```python
from build123d import *

# Parameters (mm, degrees)
BOSS_EXTRUDE1_DEPTH     = 10
CUT_EXTRUDE2_DEPTH      = 50.456381745
CUT_EXTRUDE2_DEPTH_BACK = 50.456381745
SKETCH3_R               = 2.5
CUT_EXTRUDE3_DEPTH      = 6
SKETCH4_R               = 2
CUT_REVOLVE1_ANGLE      = 90
SKETCH5_R               = 2
CUT_EXTRUDE4_DEPTH      = 2.805452299
FILLET1_R               = 5
SKETCH6_W               = 10
SKETCH6_H               = 29.685485307
CUT_EXTRUDE5_DEPTH      = 33
SKETCH7_W               = 19.76767366
SKETCH7_H               = 10
CUT_EXTRUDE6_DEPTH      = 48.418220859
SKETCH8_W               = 3.5
SKETCH8_H               = 11.210857043
CUT_EXTRUDE7_DEPTH      = 48.41822072
FILLET2_R               = 3


with BuildPart() as part:
    # Sketch1 → Boss-Extrude1 (new body)
    with BuildSketch(Plane.XY):
        with BuildLine():
            Line((0, 0), (45, 0))
            Line((45, 0), (45, 11.1125))
            Line((45, 11.1125), (35, 11.1125))
            add(Edge.make_bspline(
                [(10, 11.1125), (14.576625097, 20.181995974), (30.423374903, 20.181995974), (35, 11.1125)],
                knots=[0, 0, 0, 0, 1, 1, 1, 1], degree=3))
            Line((10, 11.1125), (0, 11.1125))
            Line((0, 11.1125), (0, 0))
        make_face()
    extrude(amount=-BOSS_EXTRUDE1_DEPTH)

    # Sketch2 → Cut-Extrude2 (cut, two sides: drawn at the far end of the back side and taken through both)
    with BuildSketch(Plane.XY.offset(-CUT_EXTRUDE2_DEPTH_BACK)):
        with BuildLine():
            Line((33, 0), (33, 10.610904597))
            add(Edge.make_bspline(
                [(33, 10.610904597), (32.518518069, 11.455367364), (31.27134268, 12.982349636), (27.931157473, 15.20113612), (22.5, 16.390279221), (17.068842527, 15.20113612), (13.72865732, 12.982349636), (12.481481931, 11.455367364), (12, 10.610904597)],
                knots=[0.018308459, 0.018308459, 0.018308459, 0.018308459, 0.138731344, 0.25915423, 0.5, 0.74084577, 0.861268656, 0.981691541, 0.981691541, 0.981691541, 0.981691541], degree=3))
            Line((12, 10.610904597), (12, 0))
            Line((12, 0), (33, 0))
        make_face()
    extrude(amount=CUT_EXTRUDE2_DEPTH + CUT_EXTRUDE2_DEPTH_BACK, mode=Mode.SUBTRACT)

    # Sketch3 → Cut-Extrude3 (cut)
    with BuildSketch(Plane(origin=(12, 0, 0), x_dir=(0, 0, -1), z_dir=(1, 0, 0))):
        with Locations(Location((5, 5.305452299, 0), (0, 0, 90))):
            Circle(SKETCH3_R)
    cut_extrude3 = extrude(amount=-CUT_EXTRUDE3_DEPTH, mode=Mode.SUBTRACT)

    # Sketch4 → Cut-Revolve1 (revolve, cut)
    with BuildSketch(Plane(origin=(6, 0, 0), x_dir=(0, 0, -1), z_dir=(1, 0, 0))):
        with Locations((5, 5.305452299)):
            Circle(SKETCH4_R)
    cut_revolve1 = revolve(axis=Axis((6, 2.805452299, -5), (0, 0, 1)), revolution_arc=CUT_REVOLVE1_ANGLE, mode=Mode.SUBTRACT)

    # Sketch5 → Cut-Extrude4 (cut)
    with BuildSketch(Plane(origin=(0, 2.805452299, 0), x_dir=(1, 0, 0), z_dir=(0, 1, 0))):
        with Locations(Location((3.5, 5, 0), (0, 0, 180))):
            Circle(SKETCH5_R)
    cut_extrude4 = extrude(amount=-CUT_EXTRUDE4_DEPTH, mode=Mode.SUBTRACT)

    # Mirror1: Cut-Extrude3, Cut-Revolve1, Cut-Extrude4 across plane
    add(cut_extrude3.mirror(Plane(origin=(22.5, 0, 0), x_dir=(0, 0, 1), z_dir=(1, 0, 0))), mode=Mode.SUBTRACT)
    add(cut_revolve1.mirror(Plane(origin=(22.5, 0, 0), x_dir=(0, 0, 1), z_dir=(1, 0, 0))), mode=Mode.SUBTRACT)
    add(cut_extrude4.mirror(Plane(origin=(22.5, 0, 0), x_dir=(0, 0, 1), z_dir=(1, 0, 0))), mode=Mode.SUBTRACT)

    # Fillet1
    fillet1_edges = [part.edges().sort_by_distance(p)[0] for p in [
        (10, 11.1125, -5),
        (35, 11.1125, -5),
        (33, 10.610904597, -5),
        (12, 10.610904597, -5),
    ]]
    fillet(fillet1_edges, radius=FILLET1_R)

    # Sketch6 → Cut-Extrude5 (cut)
    with BuildSketch(Plane.ZY):
        with Locations((-5, 14.842742654)):
            Rectangle(SKETCH6_W, SKETCH6_H)
    extrude(amount=-CUT_EXTRUDE5_DEPTH, mode=Mode.SUBTRACT)

    # Sketch7 → Cut-Extrude6 (cut, through all)
    with BuildSketch(Plane(origin=(0, 11.1125, 0), x_dir=(1, 0, 0), z_dir=(0, 1, 0))):
        with Locations((35.11616317, 5)):
            Rectangle(SKETCH7_W, SKETCH7_H)
    extrude(amount=CUT_EXTRUDE6_DEPTH, mode=Mode.SUBTRACT)

    # Sketch8 → Cut-Extrude7 (cut, through all)
    with BuildSketch(Plane.XZ):
        with Locations((43.25, -4.394571478)):
            Rectangle(SKETCH8_W, SKETCH8_H)
    extrude(amount=-CUT_EXTRUDE7_DEPTH, mode=Mode.SUBTRACT)

    # Fillet2
    # the kernel refuses this fillet: 3 mm, written as the material it takes off along each edge
    with BuildSketch(Plane(origin=(33, 18.6125, -10), x_dir=(0, 0, 1), z_dir=(0, -1, 0)), Plane(origin=(33, 18.6125, 0), x_dir=(1, 0, 0), z_dir=(0, -1, 0)), Plane(origin=(41.5, -7.5, -10), x_dir=(0, 0, 1), z_dir=(0, 1, 0))) as fillet2_piece_1:
        with BuildLine():
            CenterArc((FILLET2_R, -FILLET2_R), FILLET2_R, 90, 90)
            Line((0, -FILLET2_R), (0, 0))
            Line((0, 0), (FILLET2_R, 0))
        make_face()
    extrude(amount=26.1125, mode=Mode.SUBTRACT)
    with BuildSketch(Plane(origin=(41.5, 18.6125, 0), x_dir=(-1, 0, 0), z_dir=(0, -1, 0))) as fillet2_piece_2:
        with BuildLine():
            CenterArc((FILLET2_R, FILLET2_R), FILLET2_R, 180, 90)
            Line((0, FILLET2_R), (0, 0))
            Line((0, 0), (FILLET2_R, 0))
        make_face()
    extrude(amount=26.1125, mode=Mode.SUBTRACT)


solid = part.part
```
For this review, take the finished solid that the model builds, in its own axes (mm). A direction names the side the tool comes from. Give positions to 0.01 mm unless a question says otherwise; leave off trailing zeros. Loops run counter-clockwise (first coordinate to the right, second up) from the corner with the lowest first, then second, coordinate; pieces in that order, holes last. Notation, with made-up numbers: M 11.5,41.5 L 39.5,41.5 A14 ccw 39.5,67.5 Z; hole C -10,60 d4. An arc over 180 degrees is marked long. One line per item, written item: value. Start each with the question number.
Q1. For L1, parallel to Y at x = 34.5, z = -5; L2, parallel to Z at x = 34.75, y = 3.25; L3, parallel to Z at x = 38, y = 6, list the stretches that pass through material, from the lowest coordinate up.
Q2. Add section D-D (y = 1). Give the boundary of the cut face in (x, z), and give its area (3 significant figures).
Q3. Machinability: for faces 1 (the face through (33, 9, -5)), 2 (the face through (39.5, 1.4, -5)), 3 (the face through (39, 3, -5)), which of the approach directions +Z, -Z, +X, -X, +Y, -Y give a long, thin tool a straight path to every point of the face, cutting with its end or side? Answer none if there is none.
Q4. Draft analysis for pull direction Y (two halves, no side actions). For faces 4 (the face through (37, 6, -10)), 5 (the face through (37, 11.112, -5)), 6 (the face through (35.958, 3.463, -3.31)), state which applies: released by +Y, released by -Y, zero draft, split by the parting line, or undercut.
Q5. Add section C-C (x = 34.75). Give the boundary of the cut face in (y, z).
Q6. Add section A-A (z = -6.5). Give the boundary of the cut face in (x, y), and give its area (3 significant figures).
Q7. Add section B-B (y = 10). Give the boundary of the cut face in (x, z), and give its area (3 significant figures).
Q8. Clearance check with a flat-ended pin moving along its axis: pin 1 Ø3 at (y, z) = (5.31, -5) entering from -X. State where the tip first meets the part, or that it passes through.
Reply:
1. L1: 0 to 2.81, 7.81 to 11.11
1. L2: -9.73 to -6.42, -3.58 to -0.27
1. L3: -10 to -7.4, -2.6 to 0
2. outline: M 33,-7 A3 ccw 36,-10 L 38.5,-10 A3 ccw 41.5,-7 A2 cw 41.5,-3 A3 ccw 38.5,0 L 36,0 A3 ccw 33,-3 Z
2. area: 71.0 mm²
3. face 1: +Z, -Z, -X, +Y, -Y
3. face 2: +X, -Y
3. face 3: -X
4. face 4: zero draft
4. face 5: released by +Y
4. face 6: undercut
5. outline: M 0,-9.73 L 11.11,-9.73 L 11.11,-0.27 L 0,-0.27 Z; hole C 5.31,-5 d5
6. outline: M 33,0 L 40.18,0 L 40.18,2.81 A1.18 ccw 39,3.98 L 39,3.31 L 33,3.31 Z; M 33,7.31 L 39,7.31 L 39,6.63 A3.82 cw 41.5,5.7 L 41.5,11.11 L 33,11.11 Z
6. area: 59.0 mm²
7. outline: M 33,-7 A3 ccw 36,-10 L 38.5,-10 A3 ccw 41.5,-7 L 41.5,-3 A3 ccw 38.5,0 L 36,0 A3 ccw 33,-3 Z
7. area: 77.3 mm²
8. pin 1: x = 41.05
